Check sheet for the modelled part. Datum: model origin and axes. Units: mm. Round coordinates to 2 decimals unless told otherwise and drop trailing zeros. Loops run counter-clockwise (first coordinate to the right, second up) from the corner with the lowest first, then second, coordinate; pieces in that order, holes last. Notation, with made-up numbers: (84, 85.5) - (128, 85.5) arc R15 cw to (128, 93.5) - close; hole circle Ø8 at (-29, 76.5). An arc over 180 degrees is marked (long way). Put each result on its own line as item: value.
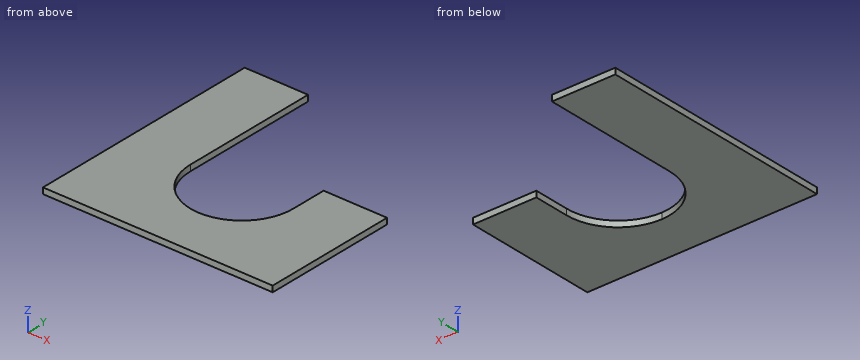
```python
from build123d import *

# Parameters (mm, degrees)
F1_DEPTH = 38.1


with BuildPart() as f1:
    # F0 (on Top) → F1 (new body)
    with BuildSketch(Plane.XY):
        with BuildLine():
            ThreePointArc((0, -330.2), (-233.486659, -233.486659), (-330.2, 0))
            Line((-330.2, 0), (-330.2, 889))
            Line((-330.2, 889), (-736.6, 889))
            Line((-736.6, 889), (-736.6, -635))
            Line((-736.6, -635), (736.6, -635))
            Line((736.6, -635), (736.6, 228.6))
            Line((736.6, 228.6), (330.2, 228.6))
            Line((330.2, 228.6), (330.2, 0))
            ThreePointArc((330.2, 0), (233.486659, -233.486659), (0, -330.2))
        make_face()
    extrude(amount=F1_DEPTH)


solid = f1.part
```
Item 1: Section check A-A on y = -187.5. Enter the section's corners in (x, z).
Filled sheet:
outline: (-736.6, 0) - (-271.8, 0) - (-271.8, 38.1) - (-736.6, 38.1) - close; (271.8, 0) - (736.6, 0) - (736.6, 38.1) - (271.8, 38.1) - close
Item 2: Go/stop test with flat-tipped pins: pin 1 (19 mm diameter, centred on x = 467.5, z = 28.5, fed in from +Y); pin 2 (2 mm diameter, centred on x = -139.5, z = 13, fed in from +Y); pin 3 (19 mm diameter, centred on y = 285.5, z = 18, fed in from +X). Record where each tip stops, or that it passes through.
Filled sheet:
pin 1: y = 228.6
pin 2: y = -298.82
pin 3: x = -330.2
Item 3: Section check D-D on x = 357. Enter the section's corners in (y, z).
Filled sheet:
outline: (-635, 0) - (228.6, 0) - (228.6, 38.1) - (-635, 38.1) - close
Item 4: Thickness scan on line 1 (X direction, y = 208.5, z = 26.5); line 2 (X direction, y = 448, z = 25); line 3 (X direction, y = -55.5, z = 27). Record the ranges inside material, lowest first. Write a range as from..to.
Filled sheet:
line 1: -736.6..-330.2, 330.2..736.6
line 2: -736.6..-330.2
line 3: -736.6..-325.5, 325.5..736.6
Item 5: Section check C-C on y = 727. Enter the section's corners in (x, z), then the cut area to 3 significant figures.
Filled sheet:
outline: (-736.6, 0) - (-330.2, 0) - (-330.2, 38.1) - (-736.6, 38.1) - close
area: 15,500 mm²
Item 6: Section check B-B on z = 8. Enter the section's corners in (x, y).
Filled sheet:
outline: (-736.6, -635) - (736.6, -635) - (736.6, 228.6) - (330.2, 228.6) - (330.2, 0) arc R330.2 cw to (0, -330.2) arc R330.2 cw to (-330.2, 0) - (-330.2, 889) - (-736.6, 889) - close
